from build123d import *

# Parameters (mm, degrees)
SKETCH1_W           = 225
SKETCH1_H           = 125
SKETCH1_W_2         = 200.2
SKETCH1_H_2         = 100.2
BOSS_EXTRUDE1_DEPTH = 1.55
SKETCH2_W           = 225
SKETCH2_H           = 125
SKETCH2_W_2         = 5
SKETCH2_H_2         = 5
BOSS_EXTRUDE2_DEPTH = 20
FILLET1_R           = 5


with BuildPart() as part:
    # Sketch1 → Boss-Extrude1 (new body)
    with BuildSketch(Plane.XY):
        with Locations((100.1, 50.1)):
            Rectangle(SKETCH1_W, SKETCH1_H)
        with Locations((100.1, 50.1)):
            Rectangle(SKETCH1_W_2, SKETCH1_H_2, mode=Mode.SUBTRACT)
    extrude(amount=BOSS_EXTRUDE1_DEPTH)

    # Sketch2 → Boss-Extrude2 (add)
    # profile 1 of 5: a face of its own
    with BuildSketch(Plane.XY.offset(1.55)):
        with Locations((100.1, 50.1)):
            Rectangle(SKETCH2_W, SKETCH2_H)
        Polygon((0, 95.2), (0, 100.2), (5, 100.2), (195.2, 100.2), (200.2, 100.2), (200.2, 95.2), (200.2, 5), (200.2, 0), (195.2, 0), (5, 0), (0, 0), (0, 5), align=None, mode=Mode.SUBTRACT)
    # profile 2 of 5: a face of its own
    with BuildSketch(Plane.XY.offset(1.55)):
        with Locations((197.7, 97.7)):
            Rectangle(SKETCH2_W_2, SKETCH2_H_2)
    # profile 3 of 5: a face of its own
    with BuildSketch(Plane.XY.offset(1.55)):
        with Locations((197.7, 2.5)):
            Rectangle(SKETCH2_W_2, SKETCH2_H_2)
    # profile 4 of 5: a face of its own
    with BuildSketch(Plane.XY.offset(1.55)):
        with Locations((2.5, 2.5)):
            Rectangle(SKETCH2_W_2, SKETCH2_H_2)
    # profile 5 of 5: a face of its own
    with BuildSketch(Plane.XY.offset(1.55)):
        with Locations((2.5, 97.7)):
            Rectangle(SKETCH2_W_2, SKETCH2_H_2)
    extrude(amount=BOSS_EXTRUDE2_DEPTH)

    # Fillet1
    fillet1_edges = [part.edges().sort_by_distance(p)[0] for p in [
        (-12.4, 112.6, 10.775),
        (212.6, 112.6, 10.775),
        (212.6, -12.4, 10.775),
        (-12.4, -12.4, 10.775),
    ]]
    fillet(fillet1_edges, radius=FILLET1_R)


solid = part.part
Work out the finished part from the listing and answer in its coordinate system (mm). A direction names the side the tool comes from. Round coordinates to 2 decimals unless told otherwise and drop trailing zeros. Loops run counter-clockwise (first coordinate to the right, second up) from the corner with the lowest first, then second, coordinate; pieces in that order, holes last. Notation, with made-up numbers: (7, 61.25) - (38, 61.25) arc R12 cw to (38, 80.25) - close; hole circle Ø11 at (0, -15). An arc over 180 degrees is marked (long way). Use one line per item in the form item = value. Start each with the question number.
(1) Find section C-C on z = 16. Determine the outline of the cut face in (x, y).
(2) Which of the six approach directions +Z, -Z, +X, -X, +Y, -Y give full straight-line access (tool end or side, diameter ignored) to faces 4 (the face through (195.2, 2, 11)), 5 (the face through (99, 112.6, 11)), 6 (the face through (198, 98, 1.55))?
(3) Determine the mould class of faces 1 (the face through (211.1, -10.97, 10.93)), 2 (the face through (99, -12.4, 11)), 3 (the face through (195.2, 98, 11)) for opening direction X: +X half, -X half, draft (parallel to the pull), parting line (faces both ways), or undercut.
(4) Find section A-A on x = 66.5. Determine the outline of the cut face in (y, z).
(5) A flat-ended cylindrical pin translates along its axis: P1, Ø1.5, axis at x = 3.5, y = 99, coming from the -Z side. Find the tip coordinate at first contact, or state that the pin passes through.
(6) Consider line 1 (X direction, y = 69, z = 2.75); line 2 (X direction, y = 97, z = 10.75); line 3 (Y direction, x = 180, z = 4.25). Determine where each line is inside the solid, lowest interval first.
(7) Find section B-B on y = 13. Determine the outline of the cut face in (x, z).
Answer list:
q1.outline = (-12.4, -7.4) arc R5 ccw to (-7.4, -12.4) - (207.6, -12.4) arc R5 ccw to (212.6, -7.4) - (212.6, 107.6) arc R5 ccw to (207.6, 112.6) - (-7.4, 112.6) arc R5 ccw to (-12.4, 107.6) - close; hole (0, 5) - (5, 5) - (5, 0) - (195.2, 0) - (195.2, 5) - (200.2, 5) - (200.2, 95.2) - (195.2, 95.2) - (195.2, 100.2) - (5, 100.2) - (5, 95.2) - (0, 95.2) - close
q2.face_4 = +Z, -Z
q2.face_5 = +Z, -Z, +X, -X, +Y
q2.face_6 = -Z
q3.face_1 = +X half
q3.face_2 = draft
q3.face_3 = undercut
q4.outline = (-12.4, 0) - (0, 0) - (0, 21.55) - (-12.4, 21.55) - close; (100.2, 0) - (112.6, 0) - (112.6, 21.55) - (100.2, 21.55) - close
q5.P1 = 1.55
q6.line_1 = -12.4 to 0, 200.2 to 212.6
q6.line_2 = -12.4 to 5, 195.2 to 212.6
q6.line_3 = -12.4 to 0, 100.2 to 112.6
q7.outline = (-12.4, 0) - (0, 0) - (0, 21.55) - (-12.4, 21.55) - close; (200.2, 0) - (212.6, 0) - (212.6, 21.55) - (200.2, 21.55) - close
